Input: part model. Units: mm. Frame: model coordinates. A direction names the side the tool comes from. Round coordinates to 2 decimals unless told otherwise and drop trailing zeros. Loops run counter-clockwise (first coordinate to the right, second up) from the corner with the lowest first, then second, coordinate; pieces in that order, holes last. Notation, with made-up numbers: (62, 47) -> (112, 47) arc R21 cw to (112, 73) -> close; hole circle Ø11 at (40.25, 45.25). An arc over 180 degrees is marked (long way). Answer in a Markdown table with one row per item. Add a question column.
Q1. Section A-A, the plane x = -15.5. Output: boundary loops of the cut face in (y, z).
Q2. Reachability of faces 1 (the face through (-7.547, -0.766, 7.383)), 2 (the face through (-17, -4, 6)), 3 (the face through (-7.547, -14.234, 7.383)), 4 (the face through (-12, -7, 16)), 5 (the face through (28, -7, 11)) from +Z, -Z, +X, -X, +Y, -Y: full face, straight path, thin tool, end or side. Return the list, or none.
Q3. Ray query, L1, parallel to Y at x = -15.5, z = 4.5; L2, parallel to X at y = -5.25, z = 3.5; L3, parallel to Z at x = 5, y = -5.75. Return the intervals inside material, ascending. Write a range as from..to.
Q4. Section C-C, the plane x = 5. Output: boundary loops of the cut face in (y, z), and give its area (3 significant figures).
Q5. Section D-D, the plane y = -4. Give the number of separate pieces and of enclosed holes in the cut face, and give its area (3 significant figures).
Q6. Section B-B, the plane z = 19.5. Output: boundary loops of the cut face in (x, y), and give its area (3 significant figures).
Q7. Pin query (flat end, axial travel): pin 1 (4 mm diameter, centred on x = 26.5, y = -11, fed in from -Z); pin 2 (4.5 mm diameter, centred on x = 26.5, y = -4, fed in from +Z); pin 3 (4.5 mm diameter, centred on y = -6, z = 17, fed in from -X); pin 4 (2.5 mm diameter, centred on x = 7.5, y = -8, fed in from -Z). Return the tip coordinate at first contact, or that it passes through.
Q8. Mould query, pull axis X, two halves, no side actions, for faces 6 (the face through (-6.434, -7.485, 6.294)), 7 (the face through (32.699, -7.395, 10.715)), 8 (the face through (-12.285, -7.605, 11.301)). Classes: pulls with the +X half, pulls with the -X half, needs draft (parallel to the pull), parting line crosses it, or undercut.
```python
from build123d import *

# Parameters (mm, degrees)
F0_R       = 2.55
F1_DEPTH   = 15
F2_R       = 4.99999
F3_R       = 1.5
F4_DEPTH   = 25
F5_R       = 1.5
F6_DEPTH   = 25
F7_SIZE2   = 3.4641016151
F7_SIZE    = 2
F7_2_SIZE2 = 3.4641016151
F7_2_SIZE  = 2
F8_R       = 11
F9_R       = 1
F10_W      = 76.274741441
F10_H      = 34.1036086902
F11_DEPTH  = 25
F12_W      = 2
F12_H      = 11
F13_DEPTH  = 15
F14_R      = 1


# Not quite as in the source:
# - a fillet or chamfer is up to 0.001 mm smaller than in the source, because OpenCascade refuses the exact size


with BuildPart() as f1:
    # F0 (on Front) → F1 (new body)
    with BuildSketch(Plane.XZ):
        Polygon((-20, 11), (-20, 0), (-20, -10), (-12, -10), (-12, -15), (23, -15), (23, -10), (31, -10), (31, 11), (23, 11), (11.7416697508, 17.5), (11.7416697508, 25.5), (-12, 25.5), (-12, 11), align=None)
        with BuildLine():
            ThreePointArc((0, -9), (-9, 0), (0, 9))
            Line((0, 9), (11, 9))
            ThreePointArc((11, 9), (20, 0), (11, -9))
            Line((11, -9), (0, -9))
        make_face(mode=Mode.SUBTRACT)
        with Locations((-6, 19.5)):
            Circle(F0_R, mode=Mode.SUBTRACT)
        with Locations((5, 19.5)):
            Circle(F0_R, mode=Mode.SUBTRACT)
    extrude(amount=F1_DEPTH)

    # F2 (radius 5 in the source; OpenCascade refuses exactly that, so slightly less here)
    f2_edges = [f1.edges().sort_by_distance(p)[0] for p in [
        (11.74167, -7.5, 25.5),
        (-12, -7.5, 25.5),
        (-12, -7.5, -15),
        (23, -7.5, -15),
        (11.74167, -7.5, 17.5),
    ]]
    fillet(f2_edges, radius=F2_R)

    # F3 (on face) → F4 (cut)
    with BuildSketch(Plane.XY.offset(11)):
        with Locations((-15.5, -4)):
            Circle(F3_R)
        with Locations((-15.5, -11)):
            Circle(F3_R)
    extrude(amount=-F4_DEPTH, mode=Mode.SUBTRACT)

    # F5 (on face) → F6 (cut)
    with BuildSketch(Plane.XY.offset(11)):
        with Locations((26.5, -4)):
            Circle(F5_R)
        with Locations((26.5, -11)):
            Circle(F5_R)
    extrude(amount=-F6_DEPTH, mode=Mode.SUBTRACT)

    # F7
    f7_edges = [f1.edges().sort_by_distance(p)[0] for p in [
        (-9, 0, 0),
        (5.5, 0, 9),
    ]]
    f7_side = f1.faces().sort_by_distance((11.090421, 0, 20.443378))[0]
    chamfer(f7_edges, length=F7_SIZE, length2=F7_SIZE2, reference=f7_side)

    # F7#2
    f7_2_edges = [f1.edges().sort_by_distance(p)[0] for p in [
        (5.5, -15, 9),
    ]]
    f7_2_side = f1.faces().sort_by_distance((11.090421, -15, 20.443378))[0]
    chamfer(f7_2_edges, length=F7_2_SIZE, length2=F7_2_SIZE2, reference=f7_2_side)

    # F8
    f8_edges = [f1.edges().sort_by_distance(p)[0] for p in [
        (-9, -11.535898, 0),
        (-9, -3.464102, 0),
        (5.5, -11.535898, 9),
        (5.5, -3.464102, 9),
    ]]
    fillet(f8_edges, radius=F8_R)

    # F9
    f9_edges = [f1.edges().sort_by_distance(p)[0] for p in [
        (-12, -7.5, 11),
        (23, -7.5, 11),
    ]]
    fillet(f9_edges, radius=F9_R)

    # F10 (on Top) → F11 (cut)
    with BuildSketch(Plane.XY):
        with Locations((3.48370336, -7.8841676004)):
            Rectangle(F10_W, F10_H)
    extrude(amount=-F11_DEPTH, mode=Mode.SUBTRACT)

    # F12 (on face) → F13 (join)
    with BuildSketch(Plane.XZ.offset(15)):
        with Locations((-21, 5.5)):
            Rectangle(F12_W, F12_H)
        with Locations((32, 5.5)):
            Rectangle(F12_W, F12_H)
    extrude(amount=-F13_DEPTH)

    # F14
    f14_edges = [f1.edges().sort_by_distance(p)[0] for p in [
        (-22, -7.5, 11),
        (33, -7.5, 11),
    ]]
    fillet(f14_edges, radius=F14_R)


solid = f1.part
```
Answer block:
| question | item | result |
|---|---|---|
| 1 | outline | (-15, 0) -> (-12.5, 0) -> (-12.5, 11) -> (-15, 11) -> close; (-9.5, 0) -> (-5.5, 0) -> (-5.5, 11) -> (-9.5, 11) -> close; (-2.5, 0) -> (0, 0) -> (0, 11) -> (-2.5, 11) -> close |
| 2 | face 1 | -Z, +Y |
| 2 | face 2 | +Z, -Z |
| 2 | face 3 | -Z, -Y |
| 2 | face 4 | +Z, -X, +Y, -Y |
| 2 | face 5 | +Z, +X, +Y, -Y |
| 3 | L1 | -15..-12.5, -9.5..-5.5, -2.5..0 |
| 3 | L2 | -22..-16.33, -14.67..-8.36, 19.36..25.67, 27.33..33 |
| 3 | L3 | 9.02..16.95, 22.05..25.5 |
| 4 | outline | (-15, 11) -> (-14.09, 10.47) arc R11 ccw to (-8.59, 9) -> (-6.41, 9) arc R11 ccw to (-0.91, 10.47) -> (0, 11) -> (0, 16.95) -> (-15, 16.95) -> close; (-15, 22.05) -> (0, 22.05) -> (0, 25.5) -> (-15, 25.5) -> close |
| 4 | area | 163 mm^2 |
| 5 | separate pieces | 3 |
| 5 | enclosed holes | 2 |
| 5 | area | 633 mm^2 |
| 6 | outline | (-12, -15) -> (-8.55, -15) -> (-8.55, 0) -> (-12, 0) -> close; (-3.45, -15) -> (2.45, -15) -> (2.45, 0) -> (-3.45, 0) -> close; (7.55, -15) -> (11.82, -15) -> (11.82, 0) -> (7.55, 0) -> close |
| 6 | area | 204 mm^2 |
| 7 | pin 1 | z = 0 |
| 7 | pin 2 | z = 11 |
| 7 | pin 3 | x = -12 |
| 7 | pin 4 | z = 9 |
| 8 | face 6 | undercut |
| 8 | face 7 | pulls with the +X half |
| 8 | face 8 | pulls with the -X half |
